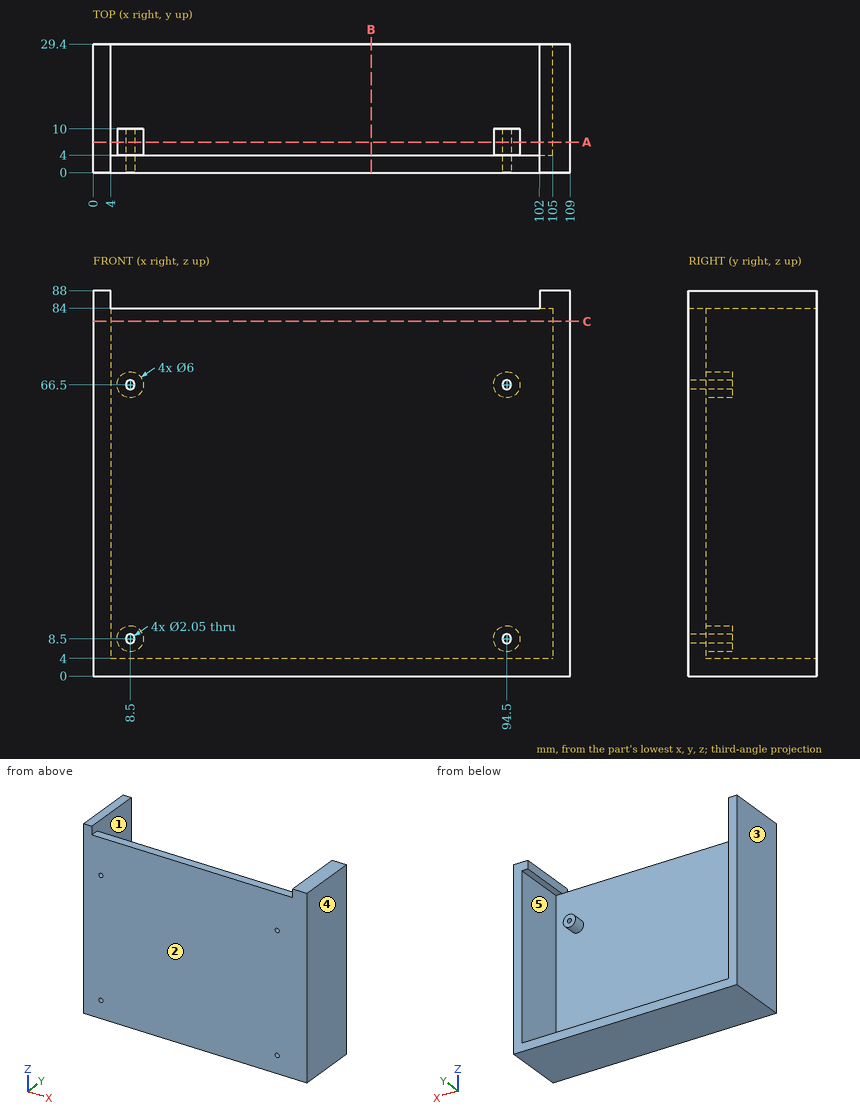
Design review of the part shown in the three views and the two pictorial views. Dimensions are in mm from the part's minimum x, y and z. A direction names the side the tool comes from. Give positions to 0.01 mm unless a question says otherwise; leave off trailing zeros. Loops run counter-clockwise (first coordinate to the right, second up) from the corner with the lowest first, then second, coordinate; pieces in that order, holes last. Notation, with made-up numbers: M 46.25,3 L 70.25,3 A14 cw 70.25,29 Z; hole C 34,83 d1. An arc over 180 degrees is marked long. Answer as a JSON object with one key per item and string values. Group by question number.
Q1. Add section C-C on z = 81. Give the boundary of the cut face in (x, y), and give its area (3 significant figures).
Q2. Mouldability with a two-part tool opening along X and no side actions: class the marked faces 1, 2 and 3 as +X half, -X half, draft (parallel to the pull), parting line (faces both ways), or undercut.
Q3. Insertion check: P1, Ø1, axis at x = 26.5, y = 8, coming from the -Z side; P2, Ø1, axis at x = 35.5, z = 50.5, coming from the +Y side; P3, Ø3.5, axis at x = 8.5, z = 8.5, coming from the +Y side; P4, Ø1.6, axis at x = 94.5, z = 8.5, coming from the +Y side. Each pin has a flat end and moves straight along its axis. Give the tip position at first contact, or say it passes through.
Q4. Add section A-A on y = 7. Give the number of separate pieces and of enclosed holes in the cut face, and give its area (3 significant figures).
Q5. Tool access review of the marked faces 4 and 5: name each direction out of +Z, -Z, +X, -X, +Y, -Y from which nothing blocks a thin tool from reaching the whole face with its end or side.
Q6. For probe 1 along X at (y, z) = (7.25, 8.5) (3 decimals); probe 2 along X at (y, z) = (25.25, 38); probe 3 along X at (y, z) = (2.75, 66.5) (3 decimals), list the stretches that pass through material, from the lowest coordinate up. Write a range as [from, to].
Q7. Add section B-B on x = 63.5. Give the boundary of the cut face in (y, z).
Checked values:
{
 "1": {"outline": "M 0,0 L 109,0 L 109,29.4 L 105,29.4 L 105,4 L 4,4 L 4,29.4 L 0,29.4 Z", "area": "639 mm²"},
 "2": {"face 1": "undercut", "face 2": "draft", "face 3": "-X half"},
 "3": {"P1": "z = 0", "P2": "y = 4", "P3": "y = 10", "P4": "through"},
 "4": {"separate pieces": "5", "enclosed holes": "4", "area": "1,220 mm²"},
 "5": {"face 4": "+Z, -Z, +X, +Y, -Y", "face 5": "+Y"},
 "6": {"probe 1": "[0, 4], [5.5, 7.475], [9.525, 11.5], [91.5, 93.475], [95.525, 97.5], [105, 109]", "probe 2": "[0, 4], [105, 109]", "probe 3": "[0, 7.475], [9.525, 93.475], [95.525, 109]"},
 "7": {"outline": "M 0,0 L 29.4,0 L 29.4,4 L 4,4 L 4,84 L 0,84 Z"}
}
